Source: CAD feature listing. Evaluate the final solid. Frame: model axes, mm. A direction names the side the tool comes from. Round coordinates to 2 decimals unless told otherwise and drop trailing zeros. Loops run counter-clockwise (first coordinate to the right, second up) from the corner with the lowest first, then second, coordinate; pieces in that order, holes last. Notation, with made-up numbers: (61.5, 53.5) -> (111.5, 53.5) arc R19 ccw to (111.5, 79.5) -> close; hole circle Ø9 at (78.5, -30). An arc over 180 degrees is marked (long way). Write item = value, one per line.
from build123d import *

# Parameters (mm, degrees)
SKETCH_4_W          = 20
SKETCH_4_H          = 20
SKETCH_4_W_2        = 15
SKETCH_4_H_2        = 15
EXTRUDE_3_DEPTH     = 60
SKETCH_5_W          = 20
SKETCH_5_H          = 30
EXTRUDE_4_DEPTH     = 10
FILLET_1_R          = 10
FILLET_2_R          = 3
FILLET_3_R          = 3
SKETCH_6_R          = 1.9
CUT_EXTRUDE_1_DEPTH = 10


with BuildPart() as part:
    # ｽｹｯﾁ4 → ﾎﾞｽ - 押し出し3 (new body)
    with BuildSketch(Plane.XY):
        Rectangle(SKETCH_4_W, SKETCH_4_H)
        Rectangle(SKETCH_4_W_2, SKETCH_4_H_2, mode=Mode.SUBTRACT)
    extrude(amount=EXTRUDE_3_DEPTH)

    # ｽｹｯﾁ5 → ﾎﾞｽ - 押し出し4 (add)
    with BuildSketch(Plane.XY):
        with Locations((0, 25)):
            Rectangle(SKETCH_5_W, SKETCH_5_H)
    extrude(amount=EXTRUDE_4_DEPTH)

    # ﾌｨﾚｯﾄ1
    fillet_1_edges = [part.edges().sort_by_distance(p)[0] for p in [
        (0, 10, 10),
    ]]
    fillet(fillet_1_edges, radius=FILLET_1_R)

    # ﾌｨﾚｯﾄ2
    fillet_2_edges = [part.edges().sort_by_distance(p)[0] for p in [
        (10, 40, 5),
        (-10, 40, 5),
        (0, 40, 10),
        (-10, 30, 10),
        (10, 30, 10),
        (10, 12.928932188, 12.928932188),
        (-10, 12.928932188, 12.928932188),
        (-10, 10, 40),
        (10, 10, 40),
    ]]
    fillet(fillet_2_edges, radius=FILLET_2_R)

    # ﾌｨﾚｯﾄ3
    fillet_3_edges = [part.edges().sort_by_distance(p)[0] for p in [
        (10, -10, 30),
        (-10, -10, 30),
    ]]
    fillet(fillet_3_edges, radius=FILLET_3_R)

    # ｽｹｯﾁ6 → ｶｯﾄ - 押し出し1 (cut)
    with BuildSketch(Plane.XY):
        with Locations((5, 25)):
            Circle(SKETCH_6_R)
        with Locations((5, 33)):
            Circle(SKETCH_6_R)
        with Locations((-5, 33)):
            Circle(SKETCH_6_R)
        with Locations((-5, 25)):
            Circle(SKETCH_6_R)
    extrude(amount=CUT_EXTRUDE_1_DEPTH, mode=Mode.SUBTRACT)


solid = part.part
1. Line query: probe 1 along Y at (x, z) = (5, 7); probe 2 along Y at (x, z) = (5.75, 34); probe 3 along X at (y, z) = (34, 7). Output: solid intervals per line, ascending. Write a range as from..to.
Evaluation:
probe_1 = -10..-7.5, 7.5..23.1, 26.9..31.1, 34.9..40
probe_2 = -10..-7.5, 7.5..10
probe_3 = -10..-6.62, -3.38..3.38, 6.62..10
2. Set-up query: faces 1 (the face through (0, 40, 3)), 2 (the face through (0, 29, 10)), 3 (the face through (0, -7.5, 30)). Return all of +Z, -Z, +X, -X, +Y, -Y with unobstructed straight access to the full face (end or side cutting, diameter ignored); none if empty.
Evaluation:
face_1 = +Z, -Z, +X, -X, +Y
face_2 = +Z, +X, -X, +Y
face_3 = +Z, -Z
3. Section query B-B (y = 25). Return the cut outline in (x, z).
Evaluation:
outline = (-10, 0) -> (-6.9, 0) -> (-6.9, 10) -> (-7, 10) arc R3 ccw to (-10, 7) -> close; (-3.1, 0) -> (3.1, 0) -> (3.1, 10) -> (-3.1, 10) -> close; (6.9, 0) -> (10, 0) -> (10, 7) arc R3 ccw to (7, 10) -> (6.9, 10) -> close
4. Contact query for flat-ended pins moving along their axis: pin 1 Ø11 at (x, y) = (-2, 27) entering from +Z; pin 2 Ø5 at (x, z) = (4.5, 23.5) entering from +Y; pin 3 Ø4.5 at (x, z) = (-2, 15.5) entering from +Y. Output: stop coordinate, or through.
Evaluation:
pin_1 = 10
pin_2 = 10
pin_3 = 12.62
5. Section query D-D (y = -4.5). Return the cut outline in (x, z).
Evaluation:
outline = (-10, 0) -> (-7.5, 0) -> (-7.5, 60) -> (-10, 60) -> close; (7.5, 0) -> (10, 0) -> (10, 60) -> (7.5, 60) -> close
6. Section query C-C (x = -0.5). Return the cut outline in (y, z), then the cut area to 3 significant figures.
Evaluation:
outline = (-10, 0) -> (-7.5, 0) -> (-7.5, 60) -> (-10, 60) -> close; (7.5, 0) -> (40, 0) -> (40, 7) arc R3 ccw to (37, 10) -> (20, 10) arc R10 cw to (10, 20) -> (10, 60) -> (7.5, 60) -> close
area = 620 mm²
7. Mould query, pull axis X, two halves, no side actions, for faces 4 (the face through (-9.14, 9.1, 39.72)), 5 (the face through (9.1, 9.14, 39.72)), 6 (the face through (-7.5, 0, 30)). Classes: released by +X, released by -X, zero draft, split by the parting line, or undercut.
Evaluation:
face_4 = released by -X
face_5 = released by +X
face_6 = undercut
8. Section query A-A (x = -5). Return the cut outline in (y, z), then the cut area to 3 significant figures.
Evaluation:
outline = (-10, 0) -> (-7.5, 0) -> (-7.5, 60) -> (-10, 60) -> close; (7.5, 0) -> (23.1, 0) -> (23.1, 10) -> (20, 10) arc R10 cw to (10, 20) -> (10, 60) -> (7.5, 60) -> close; (26.9, 0) -> (31.1, 0) -> (31.1, 10) -> (26.9, 10) -> close; (34.9, 0) -> (40, 0) -> (40, 7) arc R3 ccw to (37, 10) -> (34.9, 10) -> close
area = 544 mm²
